The model under review builds one solid part; all positions refer to its coordinate system, in mm. Face numbers are marked on the shaded views. A direction names the side the tool comes from. Coordinates: 2 decimals unless noted, no trailing zeros. Order: outer loops, then holes, each group sorted by start corner. A loop starts at its lowest first (then second) coordinate and runs counter-clockwise, first axis right, second up. Notation, with made-up numbers: (48, 87.25) -> (66, 87.25) arc R32 ccw to (66, 116.25) -> close; hole circle Ø9 at (-16, 44.25). An arc over 180 degrees is marked (long way). Answer as CSV lines item,"result". Start each with the question number.
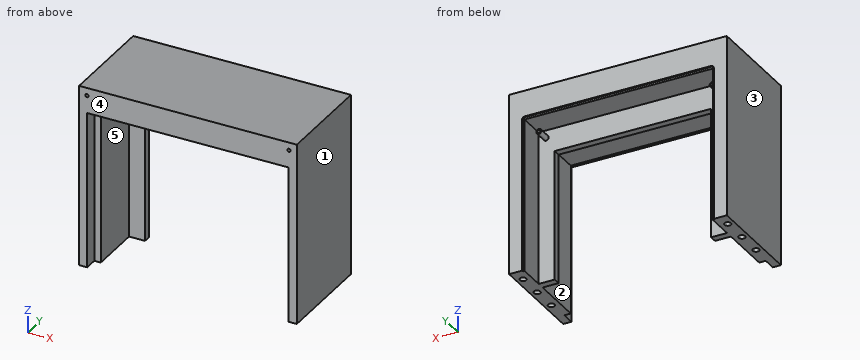
Autodesk Inventor part; units mm, degrees
ref_plane "YZ Plane" through (0, 0, 0) normal (1, 0, 0) x (0, 1, 0)
ref_plane "XZ Plane" through (0, 0, 0) normal (0, 1, 0) x (-1, 0, 0)
ref_plane "XY Plane" through (0, 0, 0) normal (0, 0, 1) x (1, 0, 0)
sketch "Sketch1" plane through (0, 0, 0) normal (0, 1, 0) x (-1, 0, 0)
  line L0 (-83.5, 139.5) -> (83.5, 139.5)
  line L1 (83.5, 139.5) -> (83.5, -139.5)
  line L2 (83.5, -139.5) -> (-83.5, -139.5)
  line L3 (-83.5, -139.5) -> (-83.5, 139.5)
  line L4 (-83.5, 139.5) -> (83.5, -139.5) construction
  line L5 (83.5, 139.5) -> (-83.5, -139.5) construction
  point P0 (0, 0)
  dimension "d0" = 167
  dimension "d1" = 279
extrude "Extrusion1" add sketch "Sketch1" along normal blind 26.6
sketch "Sketch2" plane through (0, 26.6, 0) normal (0, 1, 0) x (1, 0, 0)
  line L0 (71.5, -119.5) -> (-71.5, -119.5)
  line L1 (-73.5, -117.5) -> (-73.5, 117.5)
  line L2 (-71.5, 119.5) -> (71.5, 119.5)
  line L3 (73.5, 117.5) -> (73.5, -117.5)
  line L4 (73.5, -119.5) -> (-73.5, 119.5) construction
  line L5 (-73.5, -119.5) -> (73.5, 119.5) construction
  arc A0 (-73.5, -117.5) -> (-71.5, -119.5) centre (-71.5, -117.5) ccw
  arc A1 (-71.5, 119.5) -> (-73.5, 117.5) centre (-71.5, 117.5) ccw
  arc A2 (73.5, 117.5) -> (71.5, 119.5) centre (71.5, 117.5) ccw
  arc A3 (71.5, -119.5) -> (73.5, -117.5) centre (71.5, -117.5) ccw
  point P0 (0, 0)
  dimension "d4" = 147
  dimension "d5" = 239
  dimension "d6" = 2
extrude "Extrusion2" cut sketch "Sketch2" against normal blind 1.1
sketch "Sketch3" plane through (0, 25.5, 0) normal (0, 1, 0) x (1, 0, 0)
  line L0 (-73.5, -117.5) -> (-73.5, 117.5)
  line L1 (71.5, -119.5) -> (-71.5, -119.5)
  line L2 (-72.25, -117.83) -> (72.25, -117.83)
  line L3 (72.25, -117.83) -> (72.25, 112.27)
  line L4 (72.25, 112.27) -> (-72.25, 112.27)
  line L5 (-72.25, 112.27) -> (-72.25, -117.83)
  point P0 (0, 0)
  dimension "d9" = 1.25
  dimension "d10" = 1.67
  dimension "d11" = 144.5
  dimension "d12" = 230.1
extrude "Extrusion3" cut sketch "Sketch3" against normal blind 20
sketch "Sketch4" plane through (0, 5.5, 0) normal (0, 1, 0) x (1, 0, 0)
  circle A0 centre (-66.5, -111.83) radius 2
  line L0 (72.25, -117.83) -> (-72.25, -117.83)
  line L1 (-72.25, -117.83) -> (-72.25, 112.27)
  circle A1 centre (66.5, -111.83) radius 2
  line L2 (72.25, 112.27) -> (72.25, -117.83)
  circle A2 centre (-66.5, 106.27) radius 2
  line L3 (-72.25, 112.27) -> (72.25, 112.27)
  circle A3 centre (66.5, 106.27) radius 2
  point P0 (0, 0)
  dimension "d15" = 4
  dimension "d16" = 6
  dimension "d17" = 5.75
  dimension "d18" = 4
  dimension "d19" = 6
  dimension "d20" = 5.75
  dimension "d21" = 4
  dimension "d22" = 5.75
  dimension "d23" = 6
  dimension "d24" = 4
  dimension "d25" = 6
  dimension "d26" = 5.75
extrude "Extrusion4" add sketch "Sketch4" along normal blind 10.3 contours A0 | A1 | A2 | A3
sketch "Sketch5" plane through (0, 5.5, 0) normal (0, 1, 0) x (1, 0, 0)
  circle A0 centre (-66.5, -111.83) radius 2
  circle A1 centre (-66.5, -111.83) radius 1.25
  circle A2 centre (-66.5, 106.27) radius 2
  circle A3 centre (-66.5, 106.27) radius 1.25
  circle A4 centre (66.5, 106.27) radius 2
  circle A5 centre (66.5, 106.27) radius 1.25
  circle A6 centre (66.5, -111.83) radius 1.25
  point P0 (0, 0)
  dimension "d29" = 2.5
  dimension "d30" = 2.5
  dimension "d31" = 2.5
  dimension "d32" = 2.5
extrude "Extrusion5" cut sketch "Sketch5" along normal blind 10.3 and the other way blind 5.5 contours A1 | A3 | A5 | A6
sketch "Sketch8" plane through (0, 0, 0) normal (0, -1, 0) x (1, 0, 0)
  circle A0 centre (66.5, 111.83) radius 1.25
  circle A1 centre (66.5, 111.83) radius 1.75
  circle A2 centre (66.5, -106.27) radius 1.25
  circle A3 centre (66.5, -106.27) radius 1.75
  circle A4 centre (-66.5, -106.27) radius 1.25
  circle A5 centre (-66.5, -106.27) radius 1.75
  circle A6 centre (-66.5, 111.83) radius 1.75
  point P0 (0, 0)
  dimension "d49" = 3.5
  dimension "d50" = 3.5
  dimension "d51" = 3.5
  dimension "d52" = 3.5
extrude "Extrusion8" cut sketch "Sketch8" against normal blind 13.8
sketch "Sketch9" plane through (0, 5.5, 0) normal (0, 1, 0) x (1, 0, 0)
  line L0 (60, -100) -> (-60, -100)
  line L1 (-60, -100) -> (-60, 100)
  line L2 (-60, 100) -> (60, 100)
  line L3 (60, 100) -> (60, -100)
  line L4 (60, -100) -> (-60, 100) construction
  line L5 (-60, -100) -> (60, 100) construction
  point P0 (0, 0)
  dimension "d55" = 120
  dimension "d56" = 200
extrude "Extrusion9" cut sketch "Sketch9" against normal blind 5.8
sketch "Sketch10" plane through (0, 0, 0) normal (0, -1, 0) x (1, 0, 0)
  line L0 (83.5, 139.5) -> (83.5, -139.5)
  line L1 (-83.5, -139.5) -> (-83.5, 139.5)
  line L2 (83.5, 139.5) -> (-83.5, 139.5)
  line L3 (-83.5, 139.5) -> (-83.5, -139.5)
  line L4 (-83.5, -139.5) -> (83.5, -139.5)
  line L5 (83.5, -139.5) -> (83.5, 139.5)
  line L6 (72.25, -115.05) -> (-72.25, -115.05)
  line L7 (-72.25, -115.05) -> (-72.25, 115.05)
  line L8 (-72.25, 115.05) -> (72.25, 115.05)
  line L9 (72.25, 115.05) -> (72.25, -115.05)
  line L10 (72.25, -115.05) -> (-72.25, 115.05) construction
  line L11 (-72.25, -115.05) -> (72.25, 115.05) construction
  line L12 (-83.5, -139.5) -> (83.5, -139.5)
  line L13 (83.5, -139.5) -> (83.5, 139.5)
  line L14 (83.5, 139.5) -> (-83.5, 139.5)
  line L15 (-83.5, 139.5) -> (-83.5, -139.5)
  point P0 (0, 0)
  point P1 (71.5, 119.5)
  dimension "d67" = 144.5
  dimension "d68" = 230.1
extrude "Extrusion10" add sketch "Sketch10" along normal blind 40
sketch "Sketch12" plane through (0, -40, 0) normal (0, -1, 0) x (1, 0, 0)
  line L0 (-72.25, -115.05) -> (-72.25, 115.05)
  line L1 (72.25, -115.05) -> (-72.25, -115.05)
  line L2 (-77.25, -120.05) -> (-72.25, -120.05)
  line L3 (-72.25, -120.05) -> (-72.25, 120.05)
  line L4 (-72.25, 120.05) -> (-77.25, 120.05)
  line L5 (-77.25, 120.05) -> (-77.25, -120.05)
  line L6 (72.25, 115.05) -> (72.25, -115.05)
  line L7 (77.25, -120.05) -> (72.25, -120.05)
  line L8 (72.25, -120.05) -> (72.25, 120.05)
  line L9 (72.25, 120.05) -> (77.25, 120.05)
  line L10 (77.25, 120.05) -> (77.25, -120.05)
  line L11 (72.25, 115.05) -> (-72.25, 115.05)
  line L12 (72.25, 120.05) -> (-72.25, 120.05)
  line L13 (-72.25, 120.05) -> (-72.25, 115.05)
  line L14 (-72.25, 115.05) -> (72.25, 115.05)
  line L15 (72.25, 115.05) -> (72.25, 120.05)
  line L16 (-83.5, 139.5) -> (-83.5, -139.5)
  line L17 (83.5, 139.5) -> (-83.5, 139.5)
  line L18 (-83.5, -139.5) -> (83.5, -139.5)
  line L19 (83.5, -139.5) -> (83.5, 139.5)
  line L20 (83.5, 139.5) -> (-83.5, 139.5)
  line L21 (-83.5, 139.5) -> (-83.5, -139.5)
  line L22 (-72.25, -115.05) -> (72.25, -115.05)
  line L23 (-72.25, -115.05) -> (72.25, -115.05)
  line L24 (72.25, -115.05) -> (72.25, -120.05)
  line L25 (72.25, -120.05) -> (-72.25, -120.05)
  line L26 (-72.25, -120.05) -> (-72.25, -115.05)
  point P0 (0, 0)
  dimension "d69" = 5
  dimension "d70" = 5
  dimension "d71" = 240.1
  dimension "d72" = 5
  dimension "d73" = 5
  dimension "d74" = 240.1
extrude "Extrusion11" add sketch "Sketch12" along normal blind 10
sketch "Sketch13" plane through (0, -50, 0) normal (0, -1, 0) x (1, 0, 0)
  circle A0 centre (-77.5, -133.5) radius 1.25
  line L0 (-83.5, 139.5) -> (-83.5, -139.5)
  line L1 (-83.5, -139.5) -> (83.5, -139.5)
  circle A1 centre (-77.5, 133.5) radius 1.25
  line L2 (83.5, 139.5) -> (-83.5, 139.5)
  circle A2 centre (77.5, 133.5) radius 1.25
  line L3 (83.5, -139.5) -> (83.5, 139.5)
  circle A3 centre (77.5, -133.5) radius 1.25
  point P0 (0, 0)
  dimension "d77" = 2.5
  dimension "d78" = 6
  dimension "d79" = 6
  dimension "d80" = 2.5
  dimension "d81" = 6
  dimension "d82" = 6
  dimension "d83" = 2.5
  dimension "d84" = 6
  dimension "d85" = 6
  dimension "d86" = 6
  dimension "d87" = 6
extrude "Extrusion12" cut sketch "Sketch13" against normal blind 10 contours A0 | A1 | A2 | A3
sketch "Sketch14" plane through (83.5, 26.6, 139.5) normal (1, 0, 0) x (0, 0, -1)
  line L0 (0, 0) -> (279, 0)
  line L1 (139.5, 0) -> (139.5, -76.6)
  line L2 (259.55, -76.6) -> (19.45, -76.6)
  point P0 (139.5, -26.6)
split_face "Split1"
sketch "Sketch18" plane through (83.5, -50, 0) normal (1, 0, 0) x (0, 0, -1)
  line L0 (0, 76.6) -> (139.5, 76.6)
  line L1 (139.5, 76.6) -> (139.5, 0)
  line L2 (0, 76.6) -> (139.5, 76.6)
  line L3 (139.5, 76.6) -> (139.5, 0)
  line L4 (139.5, 0) -> (0, 0)
  line L5 (0, 0) -> (0, 76.6)
  point P0 (0, 50)
extrude "Extrusion15" cut sketch "Sketch18" against normal blind 168.1125
sketch "Sketch19" plane through (83.5, -50, 0) normal (0, 0, -1) x (-1, 0, 0)
  line L0 (0, 76.6) -> (10, 76.6)
  circle A0 centre (5, 66) radius 2.5
  circle A1 centre (5, 46) radius 2.5
  circle A2 centre (5, 26) radius 2.5
  line L1 (157, 76.6) -> (167, 76.6)
  circle A3 centre (162, 66) radius 2.5
  circle A4 centre (162, 46) radius 2.5
  circle A5 centre (162, 26) radius 2.5
  point P0 (83.5, 50)
  dimension "d97" = 5
  dimension "d99" = 5
  dimension "d101" = 5
  dimension "d102" = 5
  dimension "d104" = 5
  dimension "d106" = 5
extrude "Extrusion16" cut sketch "Sketch19" against normal blind 15
properties part number "Enclosure"
1) Wall thickness on L1, parallel to X at y = 8, z = 111.83; L2, parallel to Y at x = -78.5, z = 7.5; L3, parallel to Z at x = -66.5, y = 11.25: over which ranges is each line inside the solid? List them lowest first. Write a range as [from, to].
2) Consider section D-D (y = -4). Give the boundary of the cut face in (x, z).
3) Insertion check: pin 1 Ø2 at (x, z) = (34, 103) entering from -Y; pin 2 Ø1 at (x, z) = (-36.5, 107.5) entering from +Y; pin 3 Ø6 at (x, y) = (50, 16.5) entering from -Z. Each pin has a flat end and moves straight along its axis. Give the tip position at first contact, or say it passes through.
4) Consider section B-B (x = 24.5). Give the boundary of the cut face in (y, z).
5) Tool access review of the marked faces 1 and 2: name each direction out of +Z, -Z, +X, -X, +Y, -Y from which nothing blocks a thin tool from reaching the whole face with its end or side.
6) Mouldability with a two-part tool opening along X and no side actions: class the marked faces 3, 4 and 5 as released by +X, released by -X, zero draft, split by the parting line, or undercut.
7) Consider section C-C (y = -33.5). Give the boundary of the cut face in (x, z), plus the area to 3 significant figures.
8) Consider section A-A (z = 10). Count the separate pieces of the cut face and the enclosed holes in it, plus the area to 3 significant figures.
Result:
1,L1,"[-83.5, -72.25], [-68.5, -68.25], [-64.75, -64.5], [64.5, 64.75], [68.25, 68.5], [72.25, 83.5]"
1,L2,"[-50, -26.5], [-21.5, -6.5], [-1.5, 13.5], [18.5, 26.6]"
1,L3,"[109.83, 110.08], [113.58, 113.83], [117.83, 139.5]"
2,outline,"(-83.5, 0) -> (-81, 0) -> (-81, 15) -> (-76, 15) -> (-76, 0) -> (-72.25, 0) -> (-72.25, 115.05) -> (72.25, 115.05) -> (72.25, 0) -> (76, 0) -> (76, 15) -> (81, 15) -> (81, 0) -> (83.5, 0) -> (83.5, 139.5) -> (-83.5, 139.5) -> close"
3,pin 1,"y = 0"
3,pin 2,"y = 5.5"
3,pin 3,"z = 117.83"
4,outline,"(-50, 120.05) -> (-40, 120.05) -> (-40, 115.05) -> (0, 115.05) -> (0, 100) -> (5.5, 100) -> (5.5, 117.83) -> (25.5, 117.83) -> (25.5, 119.5) -> (26.6, 119.5) -> (26.6, 139.5) -> (-50, 139.5) -> close"
5,face 1,"+Z, -Z, +X, +Y, -Y"
5,face 2,"-Z, -Y"
6,face 3,"released by -X"
6,face 4,"zero draft"
6,face 5,"undercut"
7,outline,"(-83.5, 0) -> (-72.25, 0) -> (-72.25, 115.05) -> (72.25, 115.05) -> (72.25, 0) -> (83.5, 0) -> (83.5, 139.5) -> (-83.5, 139.5) -> close"
7,area,"6,670 mm2"
8,separate pieces,"2"
8,enclosed holes,"6"
8,area,"1,640 mm2"
